```python
from build123d import *

# Parameters (mm, degrees)
SKETCH1_W           = 150
SKETCH1_H           = 25
SKETCH1_R           = 4.05
BOSS_EXTRUDE1_DEPTH = 20
FILLET1_R           = 10
SKETCH3_R           = 1.55
CUT_EXTRUDE1_DEPTH  = 26
SKETCH3_3_R         = 3.5
SKETCH3_3_R_2       = 1.55
CUT_EXTRUDE2_DEPTH  = 3
SKETCH4_W           = 34
SKETCH4_H           = 34.075617562
CUT_EXTRUDE3_DEPTH  = 21.0000001
SKETCH5_R           = 4
CUT_EXTRUDE4_DEPTH  = 10
FILLET4_R           = 3
SKETCH6_R           = 1.55
CUT_EXTRUDE5_DEPTH  = 10
SKETCH7_W           = 2.8
SKETCH7_H           = 6
CUT_EXTRUDE6_DEPTH  = 10


with BuildPart() as part:
    # Sketch1 → Boss-Extrude1 (new body)
    with BuildSketch(Plane(origin=(0, 0, 0), x_dir=(1, 0, 0), z_dir=(0, 1, 0))):
        Rectangle(SKETCH1_W, SKETCH1_H)
        with Locations(Location((-50, 5.5, 0), (0, 0, 270))):  # turned: the seam where the file's is
            Circle(SKETCH1_R, mode=Mode.SUBTRACT)
        with Locations(Location((50, 5.5, 0), (0, 0, 270))):  # turned: the seam where the file's is
            Circle(SKETCH1_R, mode=Mode.SUBTRACT)
    extrude(amount=BOSS_EXTRUDE1_DEPTH)

    # Fillet1
    fillet1_edges = [part.edges().sort_by_distance(p)[0] for p in [
        (-75, 10, -12.5),
        (75, 10, -12.5),
    ]]
    fillet(fillet1_edges, radius=FILLET1_R)

    # Sketch3 → Cut-Extrude1 (cut, through all)
    with BuildSketch(Plane(origin=(0, 0, -12.5), x_dir=(-1, 0, 0), z_dir=(0, 0, -1))):
        with Locations((-67, 10)):
            Circle(SKETCH3_R)
        with Locations((67, 10)):
            Circle(SKETCH3_R)
    extrude(amount=-CUT_EXTRUDE1_DEPTH, mode=Mode.SUBTRACT)

    # Sketch3_3 → Cut-Extrude2 (cut)
    with BuildSketch(Plane(origin=(0, 0, -12.5), x_dir=(-1, 0, 0), z_dir=(0, 0, -1))):
        with Locations((-67, 10)):
            Circle(SKETCH3_3_R)
        with Locations((-67, 10)):
            Circle(SKETCH3_3_R_2, mode=Mode.SUBTRACT)
        with Locations((67, 10)):
            Circle(SKETCH3_3_R)
        with Locations((67, 10)):
            Circle(SKETCH3_3_R_2, mode=Mode.SUBTRACT)
    extrude(amount=-CUT_EXTRUDE2_DEPTH, mode=Mode.SUBTRACT)

    # Sketch4 → Cut-Extrude3 (cut, through all)
    with BuildSketch(Plane(origin=(0, 20, 0), x_dir=(1, 0, 0), z_dir=(0, 1, 0))):
        with Locations((0, 12.5)):
            Rectangle(SKETCH4_W, SKETCH4_H)
    extrude(amount=-CUT_EXTRUDE3_DEPTH, mode=Mode.SUBTRACT)

    # Sketch5 → Cut-Extrude4 (cut)
    with BuildSketch(Plane(origin=(0, 0, 4.537808781), x_dir=(-1, 0, 0), z_dir=(0, 0, -1))):
        with Locations((0, 10)):
            Circle(SKETCH5_R)
    extrude(amount=-CUT_EXTRUDE4_DEPTH, mode=Mode.SUBTRACT)

    # Fillet4
    fillet4_edges = [part.edges().sort_by_distance(p)[0] for p in [
        (-17, 10, 4.537808781),
        (17, 10, 4.537808781),
    ]]
    fillet(fillet4_edges, radius=FILLET4_R)

    # Sketch6 → Cut-Extrude5 (cut)
    with BuildSketch(Plane(origin=(0, 0, -12.5), x_dir=(-1, 0, 0), z_dir=(0, 0, -1))):
        with Locations((-23.5, 10)):
            Circle(SKETCH6_R)
        with Locations((23.5, 10)):
            Circle(SKETCH6_R)
    extrude(amount=-CUT_EXTRUDE5_DEPTH, mode=Mode.SUBTRACT)

    # Sketch7 → Cut-Extrude6 (cut)
    with BuildSketch(Plane.ZY.offset(-17)):
        with Locations((-9.1, 10.0294943)):
            Rectangle(SKETCH7_W, SKETCH7_H)
    cut_extrude6 = extrude(amount=-CUT_EXTRUDE6_DEPTH, mode=Mode.SUBTRACT)

    # Mirror1: Cut-Extrude6 across plane
    add(cut_extrude6.mirror(Plane(origin=(0, 0, 0), x_dir=(0, 0, 1), z_dir=(1, 0, 0))), mode=Mode.SUBTRACT)


solid = part.part
```
The listing builds one solid part. Answer for the finished solid, in the listing's coordinates (mm). A direction names the side the tool comes from. Give positions to 0.01 mm unless a question says otherwise; leave off trailing zeros. Order: outer loops, then holes, each group sorted by start corner. A loop starts at its lowest first (then second) coordinate and runs counter-clockwise, first axis right, second up. Notation, with made-up numbers: (12.25, 69) -> (46.25, 69) arc R18 cw to (46.25, 83) -> close; hole circle Ø8 at (24.25, -26.5). An arc over 180 degrees is marked (long way). Answer as a JSON object with one key per item and string values. Group by question number.
Item 1: The part is cut by section C-C on y = 1.5. Write down the section's boundary in (x, z), and give its area (3 significant figures).
Item 2: Determine the mould class of faces 1 (the flat face through (22, 11, -7.7)), 2 (the cylindrical face through (-45.984, 9.86, -6.027)) for opening direction Y: pulls with the +Y half, pulls with the -Y half, needs draft (parallel to the pull), parting line crosses it, or undercut.
Item 3: Consider L1, parallel to Y at x = 0, z = 10; L2, parallel to Y at x = 23.5, z = -11.05; L3, parallel to X at y = 11, z = -1. Determine where each line is inside the solid, lowest interval first. Write a range as from..to.
Item 4: The part is cut by section D-D on z = -5. Write down the section's boundary in (x, y), and give its area (3 significant figures).
Item 5: The part is cut by section A-A on z = 9. Write down the section's boundary in (x, y).
Item 6: The part is cut by section B-B on x = 67. Write down the section's boundary in (y, z).
Item 7: Flat-ended cylindrical pins translate along their axes: pin 1 (1.4 mm diameter, centred on y = 11.5, z = -8.5, fed in from -X); pin 2 (2 mm diameter, centred on x = -68.5, y = 8.5, fed in from -Z); pin 3 (3 mm diameter, centred on y = 9.5, z = -9.5, fed in from +X). Find the tip coordinate at first contact, or state that the pin passes through.
Item 8: A tool of negligible diameter and unlimited length cuts with its end or side. For faces 3 (the flat face through (0, 15, 4.538)), 4 (the cylindrical face through (22.068, 9.406, -11.514)), 5 (the flat face through (22, 13.029, -9)), from which of +Z, -Z, +X, -X, +Y, -Y can it reach the whole face along a straight path? Write none if from no direction.
Result set:
{
 "1": {"outline": "(-75, -2.5) arc R10 ccw to (-65, -12.5) -> (-17, -12.5) -> (-17, 1.54) arc R3 cw to (-14, 4.54) -> (14, 4.54) arc R3 cw to (17, 1.54) -> (17, -12.5) -> (65, -12.5) arc R10 ccw to (75, -2.5) -> (75, 12.5) -> (-75, 12.5) -> close; hole circle Ø8.1 at (-50, -5.5); hole circle Ø8.1 at (50, -5.5)", "area": "3,030 mm²"},
 "2": {"face 1": "undercut", "face 2": "needs draft"},
 "3": {"L1": "0..6, 14..20", "L2": "0..8.45, 11.55..20", "L3": "-75..-68.18, -65.82..-17, 17..65.82, 68.18..75"},
 "4": {"outline": "(-74.68, 0) -> (-54.02, 0) -> (-54.02, 20) -> (-74.68, 20) -> close; (-45.98, 0) -> (-17, 0) -> (-17, 20) -> (-45.98, 20) -> close; (17, 0) -> (45.98, 0) -> (45.98, 20) -> (17, 20) -> close; (54.02, 0) -> (74.68, 0) -> (74.68, 20) -> (54.02, 20) -> close; hole circle Ø3.1 at (-67, 10); hole circle Ø3.1 at (-23.5, 10); hole circle Ø3.1 at (23.5, 10); hole circle Ø3.1 at (67, 10)", "area": "1,960 mm²"},
 "5": {"outline": "(-75, 0) -> (75, 0) -> (75, 20) -> (-75, 20) -> close; hole circle Ø3.1 at (-67, 10); hole circle Ø8 at (0, 10); hole circle Ø3.1 at (67, 10)"},
 "6": {"outline": "(0, -12.3) -> (6.5, -12.3) -> (6.5, -9.5) -> (8.45, -9.5) -> (8.45, 12.5) -> (0, 12.5) -> close; (11.55, -9.5) -> (13.5, -9.5) -> (13.5, -12.3) -> (20, -12.3) -> (20, 12.5) -> (11.55, 12.5) -> close"},
 "7": {"pin 1": "x = -73.48", "pin 2": "z = -9.5", "pin 3": "x = 73.35"},
 "8": {"face 3": "-Z, +Y, -Y", "face 4": "-Z", "face 5": "none"}
}
